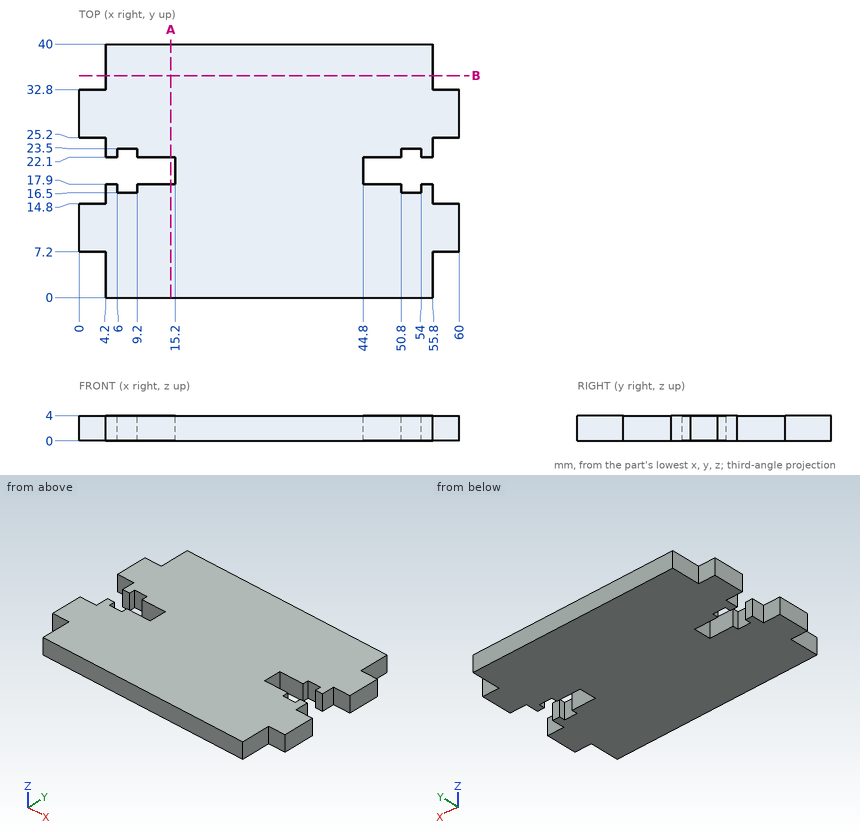
Source: three-view drawing plus pictorial views. Frame: mm from the lowest corner of the part. Coordinates: 2 decimals unless noted, no trailing zeros. Loops run counter-clockwise (first coordinate to the right, second up) from the corner with the lowest first, then second, coordinate; pieces in that order, holes last. Notation, with made-up numbers: (24, 78) - (51, 78) arc R30 ccw to (51, 113) - close; hole circle Ø6 at (18.25, 58). An arc over 180 degrees is marked (long way). Answer in a Markdown table with one row per item. Add a question column.
Item 1: Line query: line 1 along Y through (x, z) = (8, 3.1); line 2 along Y through (x, z) = (11, 1.4); line 3 along X through (y, z) = (18, 3.55). Output: solid intervals per line, ascending. Write a range as [from, to].
Item 2: Section query A-A on x = 14.5. Return the cut outline in (y, z), then the cut area to 3 significant figures.
Item 3: Contact query for flat-ended pins moving along their axis: P1, Ø1.2, axis at y = 37.5, z = 1, coming from the -X side; P2, Ø1.2, axis at y = 35.5, z = 2, coming from the +X side. Output: stop coordinate, or through.
Item 4: Section query B-B on y = 35. Return the cut outline in (x, z).
Recorded:
| question | item | result |
|---|---|---|
| 1 | line 1 | [0, 16.5], [23.5, 40] |
| 1 | line 2 | [0, 17.9], [22.1, 40] |
| 1 | line 3 | [15.2, 44.8] |
| 2 | outline | (0, 0) - (17.9, 0) - (17.9, 4) - (0, 4) - close; (22.1, 0) - (40, 0) - (40, 4) - (22.1, 4) - close |
| 2 | area | 143 mm^2 |
| 3 | P1 | x = 4.2 |
| 3 | P2 | x = 55.8 |
| 4 | outline | (4.2, 0) - (55.8, 0) - (55.8, 4) - (4.2, 4) - close |
